from build123d import *

# Parameters (mm, degrees)
SKETCH_1_W          = 110
SKETCH_1_H          = 3
EXTRUDE_1_DEPTH     = 11
SKETCH_2_W          = 136
SKETCH_2_H          = 3
EXTRUDE_2_DEPTH     = 14
SKETCH_3_W          = 136
SKETCH_3_H          = 6
EXTRUDE_3_DEPTH     = 3
SKETCH_4_W          = 130
SKETCH_4_H          = 3
EXTRUDE_4_DEPTH     = 32
CUT_EXTRUDE_1_DEPTH = 1
EXTRUDE_5_REACH     = 146.613
SKETCH_7_W          = 2.5
SKETCH_7_H          = 3
SKETCH_8_W          = 3
SKETCH_8_H          = 1.5
CUT_EXTRUDE_2_DEPTH = 2.5
SKETCH_9_W          = 3
SKETCH_9_H          = 1.5
CUT_EXTRUDE_3_DEPTH = 2.5
CUT_EXTRUDE_4_REACH = 128.174
SKETCH_10_R         = 1.3
SKETCH_11_W         = 40
SKETCH_11_H         = 11
SKETCH_11_W_2       = 16
SKETCH_11_H_2       = 3.5
CUT_EXTRUDE_5_DEPTH = 127.173778052


with BuildPart() as part:
    # 草圖1 → 填料-伸長1 (new body)
    with BuildSketch(Plane.XY):
        with Locations((-47.028571429, 0.492857143)):
            Rectangle(SKETCH_1_W, SKETCH_1_H)
    extrude(amount=EXTRUDE_1_DEPTH)

    # 草圖2 → 填料-伸長2 (add)
    with BuildSketch(Plane(origin=(0, 0, 0), x_dir=(-1, 0, 0), z_dir=(0, 0, -1))):
        with Locations((47.028571429, 0.492857143)):
            Rectangle(SKETCH_2_W, SKETCH_2_H)
    extrude(amount=EXTRUDE_2_DEPTH)

    # 草圖3 → 填料-伸長3 (add)
    with BuildSketch(Plane(origin=(0, 0, -14), x_dir=(-1, 0, 0), z_dir=(0, 0, -1))):
        with Locations((47.028571429, -1.007142857)):
            Rectangle(SKETCH_3_W, SKETCH_3_H)
    extrude(amount=EXTRUDE_3_DEPTH)

    # 草圖4 → 填料-伸長4 (add)
    with BuildSketch(Plane(origin=(0, 0, -17), x_dir=(-1, 0, 0), z_dir=(0, 0, -1))):
        Polygon((-20.971428571, -4.007142857), (115.028571429, -4.007142857), (115.028571429, -1.007142857), (112.028571429, -1.007142857), (-17.971428571, -1.007142857), (-20.971428571, -1.007142857), align=None)
        with Locations((47.028571429, 0.492857143)):
            Rectangle(SKETCH_4_W, SKETCH_4_H)
    extrude(amount=EXTRUDE_4_DEPTH)

    # 草圖5 → 除料-伸長1 (cut)
    with BuildSketch(Plane(origin=(0, 1.992857143, 0), x_dir=(1, 0, 0), z_dir=(0, 1, 0))):
        with BuildLine():
            add(Edge.make_bspline(
                [(-48.220366343, -1.911036809), (-48.270541407, -1.91028686), (-48.364344083, -1.908884824), (-48.494973246, -1.891233228), (-48.606432782, -1.864670281), (-48.697312182, -1.823968869), (-48.770960962, -1.773790726), (-48.822371595, -1.70830112), (-48.855058169, -1.631392184), (-48.858131064, -1.575902375), (-48.859717816, -1.547249089)],
                knots=[0, 0, 0, 0, 1.45873791, 2.727121924, 3.828833403, 4.779149489, 5.611735354, 6.393729658, 7.170569787, 8, 8, 8, 8], degree=3))
            add(Edge.make_bspline(
                [(-48.859717816, -1.547249089), (-48.859067643, -1.524353202), (-48.857792041, -1.479432717), (-48.848509693, -1.414107352), (-48.830269076, -1.353834434), (-48.807934617, -1.297240882), (-48.776845824, -1.245857786), (-48.73947396, -1.198744224), (-48.695811026, -1.155390258), (-48.643573446, -1.119347879), (-48.58700269, -1.084220527), (-48.522090534, -1.057366485), (-48.452126202, -1.031020798), (-48.374003189, -1.012615071), (-48.28987434, -0.995717942), (-48.198785859, -0.985465569), (-48.101387827, -0.978697318), (-48.034129185, -0.977978226), (-47.99926183, -0.977605443)],
                knots=[0, 0, 0, 0, 0.939525648, 1.843298225, 2.696554254, 3.5181456, 4.333093057, 5.149672587, 5.981863818, 6.845973329, 7.747779578, 8.708210785, 9.721263674, 10.812355027, 11.995550541, 13.240878593, 14.569652006, 16, 16, 16, 16], degree=3))
            Line((-47.99926183, -0.977605443), (-47.92192971, -0.977605443))
            add(Edge.make_bspline(
                [(-47.92192971, -0.977605443), (-47.907747598, -0.977653916), (-47.87818965, -0.977754942), (-47.848927636, -0.981955468), (-47.833705742, -0.984140552)],
                knots=[0, 0, 0, 0, 0.959614092, 2, 2, 2, 2], degree=3))
            Line((-47.833705742, -0.984140552), (-47.316342966, 2.280146269))
            add(Edge.make_bspline(
                [(-47.316342966, 2.280146269), (-47.345668471, 2.262935651), (-47.40078619, 2.230588039), (-47.480262355, 2.186880195), (-47.549909775, 2.148608363), (-47.611299516, 2.1185844), (-47.662490647, 2.093025466), (-47.706107648, 2.078035164), (-47.73968456, 2.064921848), (-47.759932978, 2.063076729), (-47.768354654, 2.062309311)],
                knots=[0, 0, 0, 0, 1.618709582, 3.042388521, 4.318437639, 5.400649213, 6.297638627, 7.036053737, 7.59907764, 8, 8, 8, 8], degree=3))
            add(Edge.make_bspline(
                [(-47.768354654, 2.062309311), (-47.798642133, 2.063656774), (-47.857249869, 2.06626418), (-47.941602172, 2.090018879), (-48.017357284, 2.13011156), (-48.08502679, 2.183226474), (-48.140088137, 2.247846893), (-48.180034599, 2.320139031), (-48.205597516, 2.397901123), (-48.208170919, 2.452041748), (-48.209474495, 2.479467086)],
                knots=[0, 0, 0, 0, 1.075146434, 2.080460303, 3.085028113, 4.105066915, 5.121505953, 6.080595913, 7.027711528, 8, 8, 8, 8], degree=3))
            add(Edge.make_bspline(
                [(-48.209474495, 2.479467086), (-48.208816812, 2.498828628), (-48.207480817, 2.538159014), (-48.190274999, 2.596456162), (-48.166994024, 2.656064112), (-48.13067359, 2.714646481), (-48.086993317, 2.775009305), (-48.033359047, 2.836236327), (-47.968905095, 2.896683711), (-47.921447851, 2.935397881), (-47.89687846, 2.95544084)],
                knots=[0, 0, 0, 0, 0.787225613, 1.599143722, 2.462777159, 3.392467032, 4.399736937, 5.501852795, 6.706668326, 8, 8, 8, 8], degree=3))
            Line((-47.89687846, 2.95544084), (-47.429618184, 3.252788288))
            Line((-47.429618184, 3.252788288), (-46.922058071, 3.608951715))
            add(Edge.make_bspline(
                [(-46.922058071, 3.608951715), (-46.876413832, 3.639138489), (-46.788094754, 3.697548226), (-46.645736231, 3.75807991), (-46.503481767, 3.798286546), (-46.407496481, 3.802782202), (-46.360038718, 3.805004978)],
                knots=[0, 0, 0, 0, 1.084242535, 2.09794932, 3.059573881, 4, 4, 4, 4], degree=3))
            add(Edge.make_bspline(
                [(-46.360038718, 3.805004978), (-46.3381608, 3.804388851), (-46.296781759, 3.803223532), (-46.239109283, 3.788739172), (-46.189869766, 3.765868881), (-46.148963408, 3.733393204), (-46.11814663, 3.690639657), (-46.096158463, 3.638981159), (-46.083357921, 3.578342667), (-46.08195108, 3.53495132), (-46.081207412, 3.512014269)],
                knots=[0, 0, 0, 0, 1.130594233, 2.138361778, 3.055019383, 3.924169546, 4.811632327, 5.75471089, 6.813120257, 8, 8, 8, 8], degree=3))
            add(Edge.make_bspline(
                [(-46.081207412, 3.512014269), (-46.08156363, 3.505479814), (-46.08243511, 3.489493395), (-46.084204273, 3.461029672), (-46.090707373, 3.424207889), (-46.09642404, 3.378657845), (-46.106005481, 3.324747731), (-46.115079801, 3.262129111), (-46.127301873, 3.191363134), (-46.14168701, 3.112256155), (-46.157847106, 3.024360372), (-46.176607518, 2.927900752), (-46.195977289, 2.822862657), (-46.217822392, 2.709597476), (-46.241950094, 2.588075039), (-46.266930873, 2.457651605), (-46.293968395, 2.318923362), (-46.313154025, 2.223498794), (-46.323006436, 2.174495345)],
                knots=[0, 0, 0, 0, 0.23106447, 0.565294867, 1.005764972, 1.549550621, 2.185906339, 2.938197749, 3.783158138, 4.720914698, 5.776755442, 6.938105291, 8.189993867, 9.547402134, 11.010355101, 12.563823371, 14.235417664, 16, 16, 16, 16], degree=3))
            add(Edge.make_bspline(
                [(-46.323006436, 2.174495345), (-46.357825146, 1.994478693), (-46.428386042, 1.629670918), (-46.529401683, 1.074537611), (-46.627786589, 0.504560358), (-46.68938042, 0.119270973), (-46.720558885, -0.075760435)],
                knots=[0, 0, 0, 0, 0.962799145, 1.951134026, 2.962875099, 4, 4, 4, 4], degree=3))
            Line((-46.720558885, -0.075760435), (-46.863242092, -0.969981149))
            Line((-46.863242092, -0.969981149), (-46.621443068, -0.969981149))
            add(Edge.make_bspline(
                [(-46.621443068, -0.969981149), (-46.590828719, -0.971065908), (-46.531735764, -0.97315975), (-46.447558792, -0.994017247), (-46.37289879, -1.030001679), (-46.307480713, -1.077598676), (-46.253676365, -1.136347365), (-46.214944889, -1.204076877), (-46.190689754, -1.279514507), (-46.188165035, -1.332490786), (-46.186858337, -1.359909305)],
                knots=[0, 0, 0, 0, 1.122867763, 2.167401115, 3.157408072, 4.149478012, 5.12172718, 6.059443137, 6.995641138, 8, 8, 8, 8], degree=3))
            add(Edge.make_bspline(
                [(-46.186858337, -1.359909305), (-46.188429675, -1.395769989), (-46.191525997, -1.466433442), (-46.225931374, -1.567887827), (-46.277285831, -1.663022499), (-46.349235784, -1.748021435), (-46.435799472, -1.820134294), (-46.535216898, -1.873541109), (-46.646458865, -1.904887272), (-46.72398679, -1.908939039), (-46.764126276, -1.911036809)],
                knots=[0, 0, 0, 0, 0.967297154, 1.906058354, 2.869352191, 3.881168242, 4.9005468, 5.90310656, 6.91434956, 8, 8, 8, 8], degree=3))
            Line((-46.764126276, -1.911036809), (-48.220366343, -1.911036809))
        make_face()
    extrude(amount=-CUT_EXTRUDE_1_DEPTH, mode=Mode.SUBTRACT)

    # 填料-伸長5: up to this face of the body (flat: up to its plane)
    extrude_5_end = Plane(part.part.faces().sort_by_distance((-115.028571429, -1.526373626, -23.980769231))[0])
    # 草圖7 → 填料-伸長5 (add, up to the picked face)
    with BuildSketch(Plane(origin=(20.971428571, 0, 0), x_dir=(0, 0, -1), z_dir=(1, 0, 0)), mode=Mode.PRIVATE) as extrude_5_sk1:
        with Locations((50.25, -1.007142857)):
            Rectangle(SKETCH_7_W, SKETCH_7_H)
    extrude_5_tool1 = split(extrude(extrude_5_sk1.sketch, amount=-EXTRUDE_5_REACH, mode=Mode.PRIVATE), bisect_by=extrude_5_end, keep=Keep.BOTH, mode=Mode.PRIVATE)
    add(extrude_5_tool1.solids().sort_by(Axis((20.971429, -1.007143, -50.25), (-1, 0, 0)))[0])

    # 草圖8 → 除料-伸長2 (cut)
    with BuildSketch(Plane.XY.offset(-49)):
        with Locations((-113.528571429, -0.257142857)):
            Rectangle(SKETCH_8_W, SKETCH_8_H)
    extrude(amount=-CUT_EXTRUDE_2_DEPTH, mode=Mode.SUBTRACT)

    # 草圖9 → 除料-伸長3 (cut)
    with BuildSketch(Plane.XY.offset(-49)):
        with Locations((19.471428571, -0.257142857)):
            Rectangle(SKETCH_9_W, SKETCH_9_H)
    extrude(amount=-CUT_EXTRUDE_3_DEPTH, mode=Mode.SUBTRACT)

    # 草圖10 → 除料-伸長4 (cut, up to next)
    with BuildSketch(Plane(origin=(0, 1.992857143, 0), x_dir=(1, 0, 0), z_dir=(0, 1, 0)), mode=Mode.PRIVATE) as cut_extrude_4_sk1:
        with Locations(Location((-107.528571429, 39, 0), (0, 0, 270))):
            Circle(SKETCH_10_R)
    cut_extrude_4_tool1 = extrude(cut_extrude_4_sk1.sketch, amount=-CUT_EXTRUDE_4_REACH, mode=Mode.PRIVATE) & part.part
    # 草圖10 → 除料-伸長4 (cut, up to next)
    with BuildSketch(Plane(origin=(0, 1.992857143, 0), x_dir=(1, 0, 0), z_dir=(0, 1, 0)), mode=Mode.PRIVATE) as cut_extrude_4_sk2:
        with Locations(Location((10.971428571, 38, 0), (0, 0, 270))):
            Circle(SKETCH_10_R)
    cut_extrude_4_tool2 = extrude(cut_extrude_4_sk2.sketch, amount=-CUT_EXTRUDE_4_REACH, mode=Mode.PRIVATE) & part.part
    add(cut_extrude_4_tool1.solids().sort_by_distance((-107.528571, 1.992857, -39))[0], mode=Mode.SUBTRACT)
    add(cut_extrude_4_tool2.solids().sort_by_distance((10.971429, 1.992857, -38))[0], mode=Mode.SUBTRACT)

    # 草圖11 → 除料-伸長5 (cut, through all)
    with BuildSketch(Plane(origin=(0, 1.992857143, 0), x_dir=(1, 0, 0), z_dir=(0, 1, 0))):
        with Locations((-85.028571429, 40)):
            Rectangle(SKETCH_11_W, SKETCH_11_H)
        with Locations((-21.028571429, 36.25)):
            Rectangle(SKETCH_11_W_2, SKETCH_11_H_2)
    extrude(amount=-CUT_EXTRUDE_5_DEPTH, mode=Mode.SUBTRACT)


solid = part.part
Can you work these out from the model? Positions are in its coordinate system, mm. A direction names the side the tool comes from. Give positions to 0.01 mm unless a question says otherwise; leave off trailing zeros. Order: outer loops, then holes, each group sorted by start corner. A loop starts at its lowest first (then second) coordinate and runs counter-clockwise, first axis right, second up. Notation, with made-up numbers: M 46.5,59.5 L 75.5,59.5 A17 cw 75.5,77.5 Z; hole C 5.5,27.5 d6. An arc over 180 degrees is marked long. Use one line per item in the form item = value. Start each with the question number.
Item 1: Will these pins go through, and if not, where does the flat tip stop? pin 1 Ø2 at (y, z) = (1, -40) entering from -X; pin 2 Ø0.9 at (x, z) = (-113.5, -32) entering from +Y; pin 3 Ø3 at (x, z) = (10.97, -38) entering from +Y; pin 4 Ø1 at (y, z) = (0, -36) entering from +X.
Item 2: For faces 4 (the flat face through (-46, 0.493, -50)), 5 (the flat face through (-65.029, -1, -40)), 6 (the flat face through (19, 1, -17)), which set-ups out of +Z, -Z, +X, -X, +Y, -Y let a thin tool reach every point of the face, with its end or its side?
Item 3: If we section it at C-C (z = -12): Write out the boundary of the cut face in (x, y), then the cut area to 3 significant figures.
Item 4: We'd pull the mould along Z, two halves only. Please class faces 1 (the flat face through (7.971, 0, 5)), 2 (the cylindrical face through (11, -1, -39.3)), 3 (the flat face through (-48, 1, 11)): +Z half, -Z half, draft (parallel to the pull), parting line (faces both ways), or undercut.
Item 5: If we section it at A-A (x = -82): Write out the boundary of the cut face in (y, z), then the cut area to 4 significant figures.
Item 6: If we section it at D-D (z = 4.5): Write out the boundary of the cut face in (x, y).
Item 7: If I drill on line 1 along X through (y, z) = (-1.5, -39); line 2 along Z through (x, y) = (-84, -3); line 3 along Z through (x, y) = (-14, 0), over which ranges is the centre line in solid material (lowest first)?
Item 8: If we section it at B-B (x = 6): Write out the boundary of the cut face in (y, z), then the cut area to 4 significant figures.
Outcome:
q1.pin_1 = -112.03
q1.pin_2 = -1.01
q1.pin_3 = 1.99
q1.pin_4 = 17.97
q2.face_4 = -Z, +X, -X, +Y
q2.face_5 = +Y, -Y
q2.face_6 = -Z, +X, +Y
q3.outline = M -115.03,-1.01 L 20.97,-1.01 L 20.97,1.99 L -115.03,1.99 Z
q3.area = 408 mm2
q4.face_1 = draft
q4.face_2 = undercut
q4.face_3 = +Z half
q5.outline = M -4.01,-49 L -2.51,-49 L -2.51,-51.5 L 0.49,-51.5 L 0.49,-49 L 1.99,-49 L 1.99,-45.5 L -4.01,-45.5 Z; M -4.01,-34.5 L 1.99,-34.5 L 1.99,11 L -1.01,11 L -1.01,-14 L -4.01,-14 Z
q5.area = 226.5 mm2
q6.outline = M -102.03,-1.01 L 7.97,-1.01 L 7.97,1.99 L -102.03,1.99 Z
q7.line_1 = -115.03 to -108.83, -106.23 to -105.03, -65.03 to 10.14, 11.8 to 20.97
q7.line_2 = -49 to -45.5, -34.5 to -14
q7.line_3 = -51.5 to -38, -34.5 to 11
q8.outline = M -4.01,-49 L -2.51,-49 L -2.51,-51.5 L 0.49,-51.5 L 0.49,-49 L 1.99,-49 L 1.99,11 L -1.01,11 L -1.01,-14 L -4.01,-14 Z
q8.area = 292.5 mm2
